Autodesk Fusion 360 part; units mm, degrees
sketch "Sketch1" plane through (0, 0, 0) normal (0, 0, 1) x (1, 0, 0)
  line L0 (8.65, -8.65) -> (-8.65, -8.65)
  line L1 (-8.65, -8.65) -> (-8.65, 8.65)
  line L2 (-8.65, 8.65) -> (8.65, 8.65)
  line L3 (8.65, 8.65) -> (8.65, -8.65)
  line L4 (8.65, -8.65) -> (-8.65, 8.65) construction
  line L5 (-8.65, -8.65) -> (8.65, 8.65) construction
  circle A0 centre (0, 0) radius 3.25
  line L6 (-8.65, 8.65) -> (8.65, 8.65)
  line L7 (8.65, 8.65) -> (8.65, 6.65)
  line L8 (8.65, 6.65) -> (-8.65, 6.65)
  line L9 (-8.65, 6.65) -> (-8.65, 8.65)
  line L10 (-8.65, -8.65) -> (8.65, -8.65)
  line L11 (8.65, -8.65) -> (8.65, -6.65)
  line L12 (8.65, -6.65) -> (-8.65, -6.65)
  line L13 (-8.65, -6.65) -> (-8.65, -8.65)
  dimension "d4" = 6.5
  dimension "d10" = 2
  dimension "d11" = 2
  dimension "d12" = 13.3
extrude "Extrude2" add sketch "Sketch1" against normal blind 12
extrude "Extrude3" add sketch "Sketch1" along normal blind 25 contours L0 L1 L3 L10 L11 L12 L13 | L1 L2 L3 L6 L7 L8 L9
fillet "Fillet1" radius 8.5 4 edges at (8.65, -7.65, 25) (-8.65, -7.65, 25) (-8.65, 7.65, 25) (8.65, 7.65, 25)
sketch "Sketch3" plane through (0, -8.65, 0) normal (0, -1, 0) x (1, 0, 0)
  arc A0 (-0.15, 25) -> (-8.65, 16.5) centre (-0.15, 16.5) ccw
  line L0 (-8.65, 16.5) -> (-8.65, -12)
  line L1 (-8.65, -12) -> (8.65, -12)
  line L2 (8.65, -12) -> (8.65, 16.5)
  arc A1 (8.65, 16.5) -> (0.15, 25) centre (0.15, 16.5) ccw
  line L3 (0.15, 25) -> (-0.15, 25)
  line L4 (-8.65, 16.5) -> (8.65, 16.5) construction
  line L5 (0, 0) -> (0, 16.5) construction
  circle A2 centre (0, 16.5) radius 2.1
  line L6 (8.65, 0) -> (-8.65, 0)
  dimension "d19" = 4.2
  dimension "d21" = 11.5
extrude "Extrude4" cut sketch "Sketch3" against normal through all contours A2
sketch "Sketch7" plane through (8.65, 0, 0) normal (1, 0, 0) x (0, 1, 0)
  line L0 (8.65, 16.5) -> (6.65, 16.5)
  line L1 (6.65, 16.5) -> (6.65, 0)
  line L2 (6.65, 0) -> (-6.65, 0)
  line L3 (-6.65, 0) -> (-6.65, 16.5)
  line L4 (-6.65, 16.5) -> (-8.65, 16.5)
  line L5 (-8.65, 16.5) -> (-8.65, -12)
  line L6 (-8.65, -12) -> (8.65, -12)
  line L7 (8.65, -12) -> (8.65, 16.5)
  line L8 (0, 0) -> (8.65, 0) construction
  line L9 (8.65, 0) -> (-8.65, -12) construction
  line L10 (5.5, -9) -> (-5.5, -9)
  line L11 (-5.5, -9) -> (-5.5, -3)
  line L12 (-5.5, -3) -> (5.5, -3)
  line L13 (5.5, -3) -> (5.5, -9)
  line L14 (5.5, -9) -> (-5.5, -3) construction
  line L15 (-5.5, -9) -> (5.5, -3) construction
  point P0 (0, -6)
  dimension "d27" = 11
  dimension "d28" = 6
extrude "Extrude5" cut sketch "Sketch7" against normal blind 15 contours L10 L11 L12 L13
fillet "Fillet2" radius 6 2 edges at (0, 6.65, 0) (0, -6.65, 0)
Geometry check sheet. Reference: the model listing, model coordinates, mm. A direction names the side the tool comes from. Round coordinates to 2 decimals unless told otherwise and drop trailing zeros. Loops run counter-clockwise (first coordinate to the right, second up) from the corner with the lowest first, then second, coordinate; pieces in that order, holes last. Notation, with made-up numbers: (48, 37) - (88, 37) arc R9 ccw to (88, 51) - close; hole circle Ø9 at (74, -2). An arc over 180 degrees is marked (long way). Answer as CSV lines item,"result".
(1) Cross-section at C-C, the plane z = -2.5. Enter the section's corners in (x, y), and give its area (3 significant figures).
Output values:
outline,"(-8.65, -8.65) - (8.65, -8.65) - (8.65, 8.65) - (-8.65, 8.65) - close; hole circle Ø6.5 at (0, 0)"
area,"266 mm²"
(2) Set-up check for faces 1 (the face through (-6.23, -7.64, 22.44)), 2 (the face through (1, -5.5, -6)), 3 (the face through (5.879, 4.939, 1.804)): record each of +Z, -Z, +X, -X, +Y, -Y from which the full face is reachable in a straight line by a thin tool's end or side.
Output values:
face 1,"+Z, -X, +Y, -Y"
face 2,"+X"
face 3,"+Z, +X, -X"
(3) Depth check by flat-ended pin: pin 1 Ø4 at (x, z) = (0, 16.5) entering from +Y; pin 2 Ø0.7 at (x, y) = (-7, 0) entering from +Z; pin 3 Ø9 at (x, y) = (1, 1.5) entering from -Z; pin 4 Ø9 at (x, y) = (1.5, 0.5) entering from +Z. Enter the tip coordinate at first touch or a pass-through.
Output values:
pin 1,"passes through"
pin 2,"stops at z = 0"
pin 3,"stops at z = -12"
pin 4,"stops at z = 1.59"
(4) Cross-section at A-A, the plane z = 10. Enter the section's corners in (x, y), and give its area (3 significant figures).
Output values:
outline,"(-8.65, -8.65) - (8.65, -8.65) - (8.65, -6.65) - (-8.65, -6.65) - close; (-8.65, 6.65) - (8.65, 6.65) - (8.65, 8.65) - (-8.65, 8.65) - close"
area,"69.2 mm²"
(5) Release check for a two-part mould opening along X. For faces 4 (the face through (1.13, 7.64, 18.27)), 5 (the face through (6, 0, 0)), 6 (the face through (6.23, -7.66, 22.44)), 7 (the face through (1.13, -7.66, 18.27)) record: released by +X, released by -X, zero draft, split by the parting line, or undercut.
Output values:
face 4,"undercut"
face 5,"zero draft"
face 6,"released by +X"
face 7,"undercut"
(6) Cross-section at B-B, the plane y = 0. Enter the section's corners in (x, z).
Output values:
outline,"(-8.65, -12) - (-3.25, -12) - (-3.25, -9) - (-6.35, -9) - (-6.35, -3) - (-3.25, -3) - (-3.25, 0) - (-8.65, 0) - close; (3.25, -12) - (8.65, -12) - (8.65, -9) - (3.25, -9) - close; (3.25, -3) - (8.65, -3) - (8.65, 0) - (3.25, 0) - close"
(7) Cross-section at D-D, the plane x = -4. Enter the section's corners in (y, z), and give its area (3 significant figures).
Output values:
outline,"(-8.65, -12) - (8.65, -12) - (8.65, 24.08) - (6.65, 24.08) - (6.65, 6) arc R6 cw to (0.65, 0) - (-0.65, 0) arc R6 cw to (-6.65, 6) - (-6.65, 24.08) - (-8.65, 24.08) - close; hole (-5.5, -9) - (5.5, -9) - (5.5, -3) - (-5.5, -3) - close"
area,"253 mm²"
(8) Material ranges on line 1 along Y through (x, z) = (6.5, 19); line 2 along Y through (x, z) = (0, -11.2); line 3 along Z through (x, y) = (0, -7.3), recorded low to high.
Output values:
line 1,"y = -8.65 to -6.65, 6.65 to 8.65"
line 2,"y = -8.65 to -3.25, 3.25 to 8.65"
line 3,"z = -12 to 14.4, 18.6 to 25"
